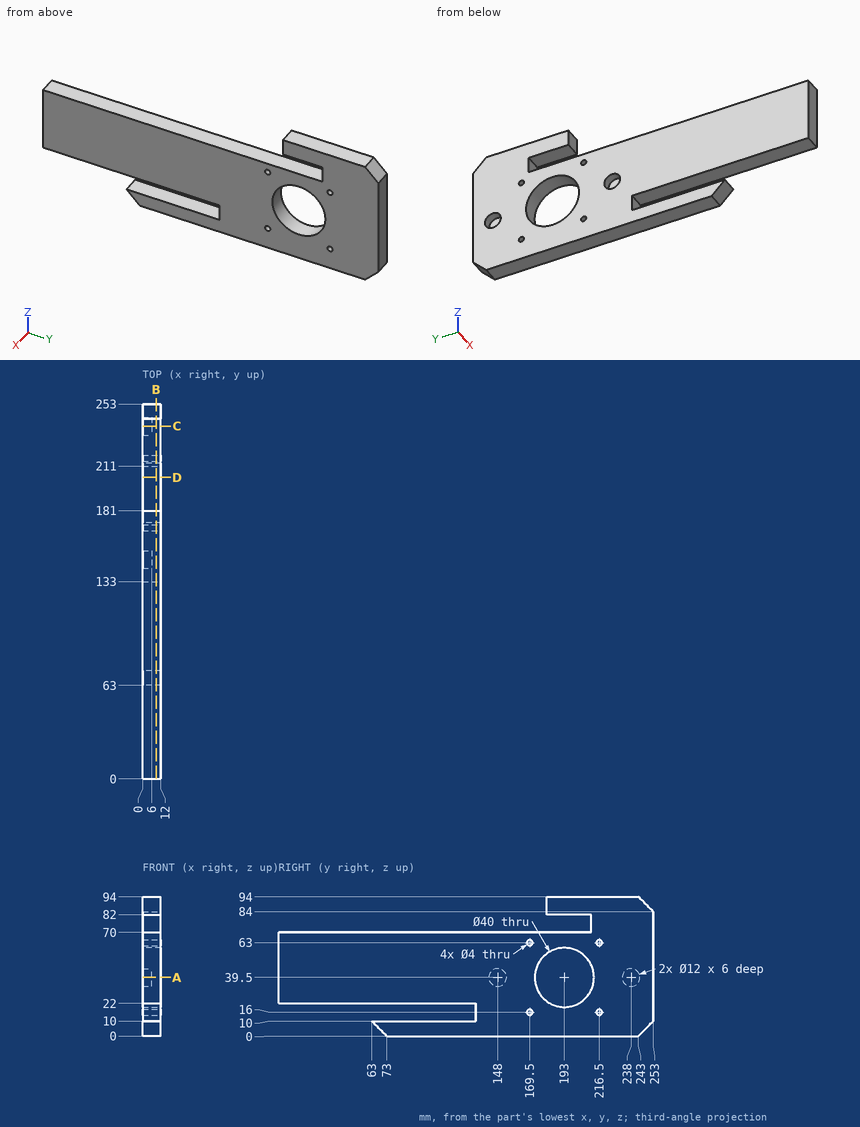
For this review, use the dimensioned drawing (mm, ordinates from the lowest corner) and the shaded views. Round coordinates to 2 decimals unless told otherwise and drop trailing zeros. Order: outer loops, then holes, each group sorted by start corner. A loop starts at its lowest first (then second) coordinate and runs counter-clockwise, first axis right, second up. Notation, with made-up numbers: M -18,75 L 1,75 A31 cw 1,103 Z; hole C 73.5,-21.5 d9. An arc over 180 degrees is marked long. Use a Markdown table: item, result. Add a question column.
Item 1: Insertion check: pin 1 (3.5 mm diameter, centred on x = 7.5, y = 81.5, fed in from +Z); pin 2 (6 mm diameter, centred on y = 150.5, z = 37, fed in from -X); pin 3 (2.5 mm diameter, centred on y = 169.5, z = 63, fed in from -X); pin 4 (6 mm diameter, centred on x = 7, z = 90.5, fed in from -Y). Each pin has a flat end and moves straight along its axis. Give the tip position at first contact, or say it passes through.
Item 2: Add section B-B, the plane x = 9. State how many separate pieces and enclosed holes the cut face has, then the cut area to 3 significant figures.
Item 3: To check wall thickness, follow line 1 along Y through (x, z) = (4.75, 39.5); line 2 along Y through (x, z) = (5.5, 63); line 3 along Z through (x, y) = (8.75, 169.5). State the ranges of each line that lie inside material, in increasing order.
Item 4: Add section D-D, the plane y = 203.5. Give the boundary of the cut face in (x, z).
Item 5: Add section A-A, the plane z = 39.5. Give the boundary of the cut face in (x, y).
Item 6: Add section C-C, the plane y = 238. Give the boundary of the cut face in (x, z).
Geometry results:
| question | item | result |
|---|---|---|
| 1 | pin 1 | stops at z = 70 |
| 1 | pin 2 | stops at x = 0 |
| 1 | pin 3 | passes through |
| 1 | pin 4 | stops at y = 181 |
| 2 | separate pieces | 1 |
| 2 | enclosed holes | 5 |
| 2 | area | 15,400 mm² |
| 3 | line 1 | y = 0 to 142, 154 to 173, 213 to 232, 244 to 253 |
| 3 | line 2 | y = 0 to 167.5, 171.5 to 214.5, 218.5 to 253 |
| 3 | line 3 | z = 0 to 14, 18 to 61, 65 to 70 |
| 4 | outline | M 0,0 L 12,0 L 12,22.48 L 0,22.48 Z; M 0,56.52 L 12,56.52 L 12,70 L 0,70 Z; M 0,82 L 12,82 L 12,94 L 0,94 Z |
| 5 | outline | M 0,0 L 12,0 L 12,173 L 0,173 L 0,154 L 6,154 L 6,142 L 0,142 Z; M 0,213 L 12,213 L 12,253 L 0,253 L 0,244 L 6,244 L 6,232 L 0,232 Z |
| 6 | outline | M 0,0 L 12,0 L 12,94 L 0,94 L 0,45.5 L 6,45.5 L 6,33.5 L 0,33.5 Z |
